Input: part model. Units: mm. Frame: model coordinates. A direction names the side the tool comes from. Give positions to 0.01 mm unless a question says otherwise; leave off trailing zeros. Loops run counter-clockwise (first coordinate to the right, second up) from the corner with the lowest first, then second, coordinate; pieces in that order, holes last. Notation, with made-up numbers: M 53,12.5 L 97,12.5 A28 cw 97,40.5 Z; hole C 49.5,16 d5. An arc over 180 degrees is marked long. Use CSV: the item, a comma, the result in double quotes. Start each with the question number.
Q1. Section C-C, the plane z = 3.25. Output: boundary loops of the cut face in (x, y).
Q2. Section B-B, the plane z = 8.5. Output: boundary loops of the cut face in (x, y), plus the area to 3 significant figures.
Q3. Section A-A, the plane z = 23.25. Output: boundary loops of the cut face in (x, y) (3 decimals).
Q4. Pin query (flat end, axial travel): pin 1 (1.4 mm diameter, centred on y = 5, z = 24.5, fed in from -X); pin 2 (2 mm diameter, centred on x = 2, y = 2.5, fed in from +Z); pin 3 (0.8 mm diameter, centred on x = -2, y = -4.5, fed in from +Z). Return the tip coordinate at first contact, or that it passes through.
Q5. Material intervals for line 1 along X through (y, z) = (0, 24.5) (3 decimals); line 2 along Z through (x, y) = (-2, 5); line 3 along Z through (x, y) = (6, -1.5), sorted ascending.
Q6. Pull-direction query (X, two-part tool) for faces 5 (the flat face through (-4, 3, 25.4)), 6 (the flat face through (0, -5, 25)), 7 (the flat face through (-5.121, 1.664, 24.774)); classes: released by +X, released by -X, zero draft, split by the parting line, or undercut.
Q7. Reachability of faces 1 (the cylindrical face through (3.787, -1.57, 12.232)), 2 (the flat face through (-2, -5, 24.13)), 3 (the flat face through (3.18, 4.38, 24.77)), 4 (the flat face through (-2, 5, 24.13)) from +Z, -Z, +X, -X, +Y, -Y: full face, straight path, thin tool, end or side. Return the list, or none.
from build123d import *

# Parameters (mm, degrees)
F3_DEPTH = 1.27
F5_DEPTH = 1.27


with BuildPart() as f1:
    # F0 (on Front) → F1 (revolve)
    with BuildSketch(Plane.XZ):
        Polygon((0, 25.4), (0, 0), (6.35, 0), (6.35, 1.27), (5.2246055566, 2.5501165073), (5.2246055566, 4.1312165558), (4.0992111132, 5.4714176804), (4.0992111132, 18.806418404), (6.35, 20.3378521087), (6.35, 25.4), align=None)
    revolve(axis=Axis((0, 0, 12.7), (0, 0, 1)))

    # F2 (on face) → F3 (cut)
    with BuildSketch(Plane.XY.offset(25.4)):
        with BuildLine():
            ThreePointArc((4.2274462149, -1.37358054), (4.3902746739, -0.6953511971), (4.445, 0))
            ThreePointArc((4.445, 0), (4.3902746739, 0.6953511971), (4.2274462149, 1.37358054))
            ThreePointArc((4.2274462149, 1.37358054), (3.59608054, 2.6127054464), (2.6127054464, 3.59608054))
            ThreePointArc((2.6127054464, 3.59608054), (1.37358054, 4.2274462149), (0, 4.445))
            ThreePointArc((0, 4.445), (-1.37358054, 4.2274462149), (-2.6127054464, 3.59608054))
            ThreePointArc((-2.6127054464, 3.59608054), (-3.59608054, 2.6127054464), (-4.2274462149, 1.37358054))
            ThreePointArc((-4.2274462149, 1.37358054), (-4.445, 0), (-4.2274462149, -1.37358054))
            ThreePointArc((-4.2274462149, -1.37358054), (-3.59608054, -2.6127054464), (-2.6127054464, -3.59608054))
            ThreePointArc((-2.6127054464, -3.59608054), (-1.37358054, -4.2274462149), (0, -4.445))
            ThreePointArc((0, -4.445), (1.37358054, -4.2274462149), (2.6127054464, -3.59608054))
            ThreePointArc((2.6127054464, -3.59608054), (3.59608054, -2.6127054464), (4.2274462149, -1.37358054))
        make_face()
        with BuildLine():
            ThreePointArc((-2.6127054464, 3.59608054), (-1.37358054, 4.2274462149), (0, 4.445))
            Line((0, 4.445), (0, 6.35))
            ThreePointArc((0, 6.35), (-1.9622579143, 6.0392088785), (-3.7324363521, 5.1372579143))
            Line((-3.7324363521, 5.1372579143), (-2.6127054464, 3.59608054))
        make_face()
        with BuildLine():
            ThreePointArc((2.6127054464, 3.59608054), (3.59608054, 2.6127054464), (4.2274462149, 1.37358054))
            Line((4.2274462149, 1.37358054), (6.0392088785, 1.9622579143))
            ThreePointArc((6.0392088785, 1.9622579143), (5.1372579143, 3.7324363521), (3.7324363521, 5.1372579143))
            Line((3.7324363521, 5.1372579143), (2.6127054464, 3.59608054))
        make_face()
        with BuildLine():
            Line((6.0392088785, -1.9622579143), (4.2274462149, -1.37358054))
            ThreePointArc((4.2274462149, -1.37358054), (3.59608054, -2.6127054464), (2.6127054464, -3.59608054))
            Line((2.6127054464, -3.59608054), (3.7324363521, -5.1372579143))
            ThreePointArc((3.7324363521, -5.1372579143), (5.1372579143, -3.7324363521), (6.0392088785, -1.9622579143))
        make_face()
        with BuildLine():
            Line((0, -6.35), (0, -4.445))
            ThreePointArc((0, -4.445), (-1.37358054, -4.2274462149), (-2.6127054464, -3.59608054))
            Line((-2.6127054464, -3.59608054), (-3.7324363521, -5.1372579143))
            ThreePointArc((-3.7324363521, -5.1372579143), (-1.9622579143, -6.0392088785), (0, -6.35))
        make_face()
        with BuildLine():
            ThreePointArc((-4.2274462149, -1.37358054), (-4.445, 0), (-4.2274462149, 1.37358054))
            Line((-4.2274462149, 1.37358054), (-6.0392088785, 1.9622579143))
            ThreePointArc((-6.0392088785, 1.9622579143), (-6.35, 0), (-6.0392088785, -1.9622579143))
            Line((-6.0392088785, -1.9622579143), (-4.2274462149, -1.37358054))
        make_face()
    extrude(amount=-F3_DEPTH, mode=Mode.SUBTRACT)

    # F4 (on face) → F5 (cut)
    with BuildSketch(Plane.XY.offset(24.13)):
        with BuildLine():
            ThreePointArc((4.2274462149, -1.37358054), (4.3902746739, -0.6953511971), (4.445, 0))
            ThreePointArc((4.445, 0), (4.3902746739, 0.6953511971), (4.2274462149, 1.37358054))
            ThreePointArc((4.2274462149, 1.37358054), (3.59608054, 2.6127054464), (2.6127054464, 3.59608054))
            ThreePointArc((2.6127054464, 3.59608054), (1.37358054, 4.2274462149), (0, 4.445))
            ThreePointArc((0, 4.445), (-1.37358054, 4.2274462149), (-2.6127054464, 3.59608054))
            ThreePointArc((-2.6127054464, 3.59608054), (-3.59608054, 2.6127054464), (-4.2274462149, 1.37358054))
            ThreePointArc((-4.2274462149, 1.37358054), (-4.445, 0), (-4.2274462149, -1.37358054))
            ThreePointArc((-4.2274462149, -1.37358054), (-3.59608054, -2.6127054464), (-2.6127054464, -3.59608054))
            ThreePointArc((-2.6127054464, -3.59608054), (-1.37358054, -4.2274462149), (0, -4.445))
            ThreePointArc((0, -4.445), (1.37358054, -4.2274462149), (2.6127054464, -3.59608054))
            ThreePointArc((2.6127054464, -3.59608054), (3.59608054, -2.6127054464), (4.2274462149, -1.37358054))
        make_face()
    extrude(amount=-F5_DEPTH, mode=Mode.SUBTRACT)


solid = f1.part
A:
1,outline,"C 0,0 d10.45"
2,outline,"C 0,0 d8.2"
2,area,"52.8 mm^2"
3,outline,"C 0,0 d12.7; hole C 0,0 d8.89"
4,pin 1,"x = -4.67"
4,pin 2,"z = 22.86"
4,pin 3,"z = 24.13"
5,line 1,"4.445 to 6.35"
5,line 2,"0 to 2.37, 19.68 to 24.13"
5,line 3,"0 to 1.46, 20.23 to 25.4"
6,face 5,"zero draft"
6,face 6,"undercut"
6,face 7,"released by -X"
7,face 1,"none"
7,face 2,"+Z, -Y"
7,face 3,"+Z, +X"
7,face 4,"+Z, +Y"
